```python
from build123d import *

# Parameters (mm, degrees)
SKETCH_W          = 22
SKETCH_H          = 10
PAD_DEPTH         = 2
SKETCH001_R       = 1.5
POCKET_DEPTH      = 2.001
POCKET_DEPTH_BACK = -0.001
SKETCH002_W       = 22
SKETCH002_H       = 10
PAD001_DEPTH      = 2
SKETCH003_R       = 1.375
POCKET001_DEPTH   = 2.001
PAD002_DEPTH      = 2
POCKET002_DEPTH   = 10.001
PAD003_DEPTH      = 24
SKETCH007_W       = 20
SKETCH007_H       = 8
POCKET003_DEPTH   = 48.001


with BuildPart() as part:
    # Sketch → Pad (new body)
    with BuildSketch(Plane.YZ):
        with Locations((1, 5)):
            Rectangle(SKETCH_W, SKETCH_H)
    extrude(amount=-PAD_DEPTH)

    # Sketch001 → Pocket (cut, two sides)
    with BuildSketch(Plane.YZ) as pocket_sk:
        with Locations((-5, 5)):
            Circle(SKETCH001_R)
    extrude(amount=-POCKET_DEPTH, mode=Mode.SUBTRACT)
    extrude(pocket_sk.sketch, amount=-POCKET_DEPTH_BACK, mode=Mode.SUBTRACT)

    # Sketch002 → Pad001 (join)
    with BuildSketch(Plane.YZ):
        with Locations((23, 5)):
            Rectangle(SKETCH002_W, SKETCH002_H)
    extrude(amount=-PAD001_DEPTH)

    # Sketch003 → Pocket001 (cut, through all)
    with BuildSketch(Plane.YZ):
        with Locations((29, 5)):
            Circle(SKETCH003_R)
    extrude(amount=-POCKET001_DEPTH, mode=Mode.SUBTRACT)

    # Sketch004 → Pad002 (join)
    with BuildSketch(Plane.XY):
        with BuildLine():
            ThreePointArc((36, 0), (48, 12), (36, 24))
            Line((36, 24), (-2, 24))
            Line((-2, 24), (-2, 0))
            Line((36, 0), (-2, 0))
        make_face()
    extrude(amount=PAD002_DEPTH)

    # Sketch005 → Pocket002 (cut, through all)
    with BuildSketch(Plane.XY):
        with BuildLine():
            ThreePointArc((2, 13.5), (0.5, 12), (2, 10.5))
            Line((2, 10.5), (44, 10.5))
            ThreePointArc((44, 10.5), (45.5, 12), (44, 13.5))
            Line((2, 13.5), (44, 13.5))
        make_face()
    extrude(amount=POCKET002_DEPTH, mode=Mode.SUBTRACT)

    # Sketch006 → Pad003 (join)
    with BuildSketch(Plane.XZ):
        Polygon((0, 10), (36, 2), (0, 2), align=None)
    extrude(amount=-PAD003_DEPTH)

    # Sketch007 → Pocket003 (cut, through all)
    with BuildSketch(Plane.YZ):
        with Locations((12, 6)):
            Rectangle(SKETCH007_W, SKETCH007_H)
    extrude(amount=POCKET003_DEPTH, mode=Mode.SUBTRACT)


solid = part.part
```
Geometry check sheet. Reference: the model listing, model coordinates, mm. A direction names the side the tool comes from. Give positions to 0.01 mm unless a question says otherwise; leave off trailing zeros. Order: outer loops, then holes, each group sorted by start corner. A loop starts at its lowest first (then second) coordinate and runs counter-clockwise, first axis right, second up. Notation, with made-up numbers: (-29.75, 78.5) - (-25.75, 78.5) arc R9 ccw to (-25.75, 82.5) - close; hole circle Ø3 at (36, -37). An arc over 180 degrees is marked (long way). Write item = value, one per line. Start each with the question number.
1) Access from +Z, -Z, +X, -X, +Y, -Y to the whole of each face (thin tool, end or side, straight path). Record for faces 4 (the flat face through (14, 0, 4)), 5 (the cylindrical face through (45.5, 12, 1)), 6 (the flat face through (24, 10, 2)), 7 (the flat face through (0, 30, 6.2)), 8 (the flat face through (-2, 12, 5)).
2) Section check A-A (y = 29). Enter the section's corners in (x, z) (3 decimals).
3) Section check B-B (x = 31.5). Enter the section's corners in (y, z).
4) Gauge pin test, flat ends, axial feed: pin 1 Ø1.6 at (x, z) = (16.5, 1.5) entering from -Y; pin 2 Ø5 at (y, z) = (-6.5, 3) entering from +X; pin 3 Ø4 at (y, z) = (24, 2) entering from +X. Record the tip position at first contact, or that the pin passes through.
5) Section check D-D (y = 12). Enter the section's corners in (x, z), then the cut area to 3 significant figures.
6) Draft check along Y on faces 1 (the cylindrical face through (48, 12, 1)), 2 (the flat face through (14, 24, 4)), 3 (the flat face through (14, 2, 5)). Enter one of: released by +Y, released by -Y, zero draft, split by the parting line, or undercut.
7) Section check C-C (z = 1.25). Enter the section's corners in (x, y).
8) Scan lines: L1, parallel to Y at x = 30, z = 1.5; L2, parallel to Y at x = 17, z = 2.5; L3, parallel to Z at x = -1.45, y = -5. Record each from-to range of solid material in increasing order.
Geometry check:
q1.face_4 = +Z, -Z, +X, -Y
q1.face_5 = +Z, -Z
q1.face_6 = +Z, +X
q1.face_7 = +Z, -Z, +X, +Y
q1.face_8 = +Z, -Z, -X, +Y, -Y
q2.outline = (-2, 0) - (0, 0) - (0, 3.625) - (-2, 3.625) - close; (-2, 6.375) - (0, 6.375) - (0, 10) - (-2, 10) - close
q3.outline = (0, 0) - (10.5, 0) - (10.5, 2) - (2, 2) - (2, 3) - (0, 3) - close; (13.5, 0) - (24, 0) - (24, 3) - (22, 3) - (22, 2) - (13.5, 2) - close
q4.pin_1 = 0
q4.pin_2 = 0
q4.pin_3 = 42.63
q5.outline = (-2, 0) - (0.5, 0) - (0.5, 2) - (0, 2) - (0, 10) - (-2, 10) - close; (45.5, 0) - (48, 0) - (48, 2) - (45.5, 2) - close
q5.area = 26.0 mm2
q6.face_1 = split by the parting line
q6.face_2 = released by +Y
q6.face_3 = undercut
q7.outline = (-2, -10) - (0, -10) - (0, 0) - (36, 0) arc R12 ccw to (36, 24) - (0, 24) - (0, 34) - (-2, 34) - close; hole (2, 10.5) - (44, 10.5) arc R1.5 ccw to (44, 13.5) - (2, 13.5) arc R1.5 ccw to start
q8.L1 = 0 to 10.5, 13.5 to 24
q8.L2 = 0 to 2, 22 to 24
q8.L3 = 0 to 3.5, 6.5 to 10
